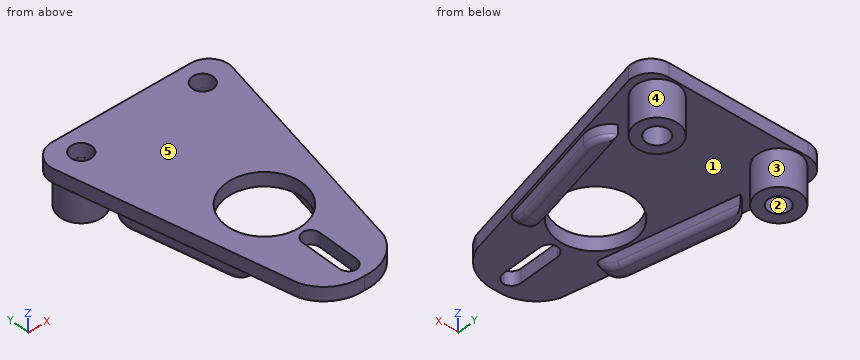
```python
from build123d import *

# Parameters (mm, degrees)
F0_W        = 3.7012519315
F0_H        = 12.7320559695
F0_R        = 8.100129487
F0_R_2      = 2.25
F1_DEPTH    = 3
F2_T1_DEPTH = 3
F3_R        = 4.5649895604
F3_R_2      = 2.4116141927
F3_R_3      = 2.2420485947
F4_DEPTH    = 8
F6_DEPTH    = 3
F7_T1_DEPTH = 14.95289459
F7_T3_DEPTH = 26.4498235383
F7_T5_DEPTH = 26.4498235383
F8_R        = 1


# Not quite as in the source:
# - a fillet or chamfer that OpenCascade refuses, or shapes differently, is made with other operations: its cross-section is extruded or revolved along the edge and cut away or added


with BuildPart() as f1:
    # F0 (on Top) → F1 (new body)
    with BuildSketch(Plane.XY):
        with BuildLine():
            Line((14.8444259539, 34.1621562839), (0, 34.1621562839))
            Line((0, 34.1621562839), (-14.8444259539, 34.1621562839))
            ThreePointArc((-14.8444259539, 34.1621562839), (-18.1303110964, 32.6596806941), (-19.1433615983, 29.1915107518))
            Line((-19.1433615983, 29.1915107518), (-9.0677291155, -18.3654725552))
            ThreePointArc((-9.0677291155, -18.3654725552), (-5.4543132889, -22.6555173257), (0, -23.9638462663))
            ThreePointArc((0, -23.9638462663), (5.4543132889, -22.6555173257), (9.0677291155, -18.3654725552))
            Line((9.0677291155, -18.3654725552), (19.1433615983, 29.1915107518))
            ThreePointArc((19.1433615983, 29.1915107518), (18.1303110964, 32.6596806941), (14.8444259539, 34.1621562839))
        make_face()
        with Locations((0, -15.5778131448)):
            Rectangle(F0_W, F0_H, mode=Mode.SUBTRACT)
        Circle(F0_R, mode=Mode.SUBTRACT)
        with Locations((-13, 29.2403830344)):
            Circle(F0_R_2, mode=Mode.SUBTRACT)
        with Locations((13, 29.2403830344)):
            Circle(F0_R_2, mode=Mode.SUBTRACT)
    extrude(amount=F1_DEPTH)

    # F2: fillet of radius 2 on 4 edges, made by hand

    # F2_s2 → F2_t1 (join)
    with BuildSketch(Plane.XY):
        with BuildLine():
            ThreePointArc((0.1493740343, -9.21178516), (-1.2648395281, -9.7975715976), (-1.8506259657, -11.21178516))
            Line((-1.8506259657, -11.21178516), (-1.8506259657, -9.21178516))
            Line((-1.8506259657, -9.21178516), (0.1493740343, -9.21178516))
        make_face()
        with BuildLine():
            ThreePointArc((1.8506259657, -11.21178516), (1.2648395281, -9.7975715976), (-0.1493740343, -9.21178516))
            Line((-0.1493740343, -9.21178516), (1.8506259657, -9.21178516))
            Line((1.8506259657, -9.21178516), (1.8506259657, -11.21178516))
        make_face()
        with BuildLine():
            ThreePointArc((-1.8506259657, -19.9438411295), (-1.2648395281, -21.3580546919), (0.1493740343, -21.9438411295))
            Line((0.1493740343, -21.9438411295), (-1.8506259657, -21.9438411295))
            Line((-1.8506259657, -21.9438411295), (-1.8506259657, -19.9438411295))
        make_face()
        with BuildLine():
            ThreePointArc((1.8506259657, -19.9438411295), (1.2648395281, -21.3580546919), (-0.1493740343, -21.9438411295))
            Line((-0.1493740343, -21.9438411295), (1.8506259657, -21.9438411295))
            Line((1.8506259657, -21.9438411295), (1.8506259657, -19.9438411295))
        make_face()
    extrude(amount=F2_T1_DEPTH)

    # F3 (on face) → F4 (join)
    with BuildSketch(Plane(origin=(0, 0, 0), x_dir=(1, 0, 0), z_dir=(0, 0, -1))):
        with Locations((13, -29.2403830344)):
            Circle(F3_R)
        with Locations((13, -29.2403830344)):
            Circle(F3_R_2, mode=Mode.SUBTRACT)
        with Locations((-13, -29.2403830344)):
            Circle(F3_R)
        with Locations((-13, -29.2403830344)):
            Circle(F3_R_3, mode=Mode.SUBTRACT)
    extrude(amount=F4_DEPTH)

    # F5 (on face) → F6 (join)
    with BuildSketch(Plane(origin=(0, 0, 0), x_dir=(1, 0, 0), z_dir=(0, 0, -1))):
        Polygon((-7.118105705, 8.1281888095), (-10.5773922314, 8.8652892849), (-16.5612712118, -19.2176554765), (-13.1019846854, -19.9547559519), align=None)
        Polygon((16.5612712118, -19.2176554765), (10.5773922314, 8.8652892849), (7.118105705, 8.1281888095), (13.1019846854, -19.9547559519), align=None)
    extrude(amount=F6_DEPTH)

    # F7: fillet of radius 5 on 4 edges, made by hand

    # F7_s2 → F7_t1 (cut)
    with BuildSketch(Plane.XY.offset(-14.95289459)):
        with BuildLine():
            ThreePointArc((-13.1019846854, 19.9547559519), (-15.2257590624, 17.6540998095), (-15.5648763993, 14.5414745957))
            Line((-15.5648763993, 14.5414745957), (-16.5612712118, 19.2176554765))
            Line((-16.5612712118, 19.2176554765), (-13.1019846854, 19.9547559519))
        make_face()
        with BuildLine():
            ThreePointArc((15.5648763993, 14.5414745957), (15.2257590624, 17.6540998095), (13.1019846854, 19.9547559519))
            Line((13.1019846854, 19.9547559519), (16.5612712118, 19.2176554765))
            Line((16.5612712118, 19.2176554765), (15.5648763993, 14.5414745957))
        make_face()
    extrude(amount=F7_T1_DEPTH, mode=Mode.SUBTRACT)

    # F7_s4 → F7_t3 (cut)
    with BuildSketch(Plane(origin=(23.1298700172, -4.9284839674, 0), x_dir=(0, 0, 1), z_dir=(-0.9780436123, 0.2084003178, 0))):
        with BuildLine():
            ThreePointArc((0, -6.4663076535), (-2.1833001327, -4.622344746), (-3, -1.8837319585))
            Line((-3, -1.8837319585), (-3, -6.4663076535))
            Line((-3, -6.4663076535), (0, -6.4663076535))
        make_face()
    extrude(amount=F7_T3_DEPTH, mode=Mode.SUBTRACT)

    # F7_s6 → F7_t5 (cut)
    with BuildSketch(Plane(origin=(2.7392109406, 0.5836676641, 0), x_dir=(0, 0, 1), z_dir=(-0.9780436123, -0.2084003178, 0))):
        with BuildLine():
            ThreePointArc((0, -6.4663076535), (-2.1833001327, -4.622344746), (-3, -1.8837319585))
            Line((-3, -1.8837319585), (-3, -6.4663076535))
            Line((-3, -6.4663076535), (0, -6.4663076535))
        make_face()
    extrude(amount=F7_T5_DEPTH, mode=Mode.SUBTRACT)

    # F8
    f8_edges = [f1.edges().sort_by_distance(p)[0] for p in [
        (-10.58755, 8.154263, -3),
        (10.58755, 8.154263, -3),
        (13.548639, 5.079072, -3),
        (-13.548639, 5.079072, -3),
        (-15.225759, 17.6541, -3),
        (-10.961675, -7.061813, -2.1833),
        (-7.502388, -6.324713, -2.1833),
        (15.225759, 17.6541, -3),
        (7.502388, -6.324713, -2.1833),
        (10.961675, -7.061813, -2.1833),
    ]]
    fillet(f8_edges, radius=F8_R)


solid = f1.part
```
Geometry check sheet. Reference: the model listing, model coordinates, mm. Face numbers are marked on the shaded views. A direction names the side the tool comes from. Coordinates: 2 decimals unless noted, no trailing zeros. Order: outer loops, then holes, each group sorted by start corner. A loop starts at its lowest first (then second) coordinate and runs counter-clockwise, first axis right, second up. Notation, with made-up numbers: M 6.5,19 L 47.5,19 A20 cw 47.5,56 Z; hole C -33.5,17.5 d7. An arc over 180 degrees is marked long. One line per question, with ' | ' between items. Start each with the question number.
Item 1: Draft check along X on the marked faces 3, 4 and 5. Enter one of: pulls with the +X half, pulls with the -X half, needs draft (parallel to the pull), parting line crosses it, or undercut.
Item 2: Gauge pin test, flat ends, axial feed: pin 1 (2 mm diameter, centred on y = 12.5, z = -5.5, fed in from +X); pin 2 (1.7 mm diameter, centred on x = -12.5, y = 3.5, fed in from -Z); pin 3 (4 mm diameter, centred on x = -14.5, z = -7, fed in from -Y); pin 4 (2.5 mm diameter, centred on y = -13.5, z = 2, fed in from -X). Record the tip position at first contact, or that the pin passes through.
Item 3: Cross-section at A-A on y = -14.5. Enter the section's corners in (x, z).
Item 4: Cross-section at B-B on z = -5.5. Enter the section's corners in (x, y), then the cut area to 3 significant figures.
Item 5: Set-up check for the marked faces 1 and 2: record each of +Z, -Z, +X, -X, +Y, -Y from which the full face is reachable in a straight line by a thin tool's end or side.
Item 6: Material ranges on L1, parallel to Y at x = -13, z = -4.25; L2, parallel to Z at x = -12.5, y = 13; L3, parallel to Z at x = 0, y = 24.5, recorded low to high. Write a range as [from, to].
Findings:
1) face 3: undercut | face 4: undercut | face 5: needs draft
2) pin 1: passes through | pin 2: stops at z = -3 | pin 3: stops at y = 24.68 | pin 4: stops at x = -10.36
3) outline: M -9.89,0 L -1.85,0 L -1.85,3 L -9.89,3 Z; M 1.85,0 L 9.89,0 L 9.89,3 L 1.85,3 Z
4) outline: C -13,29.24 d9.13; C 13,29.24 d9.13; hole C -13,29.24 d4.48; hole C 13,29.24 d4.82 | area: 96.9 mm²
5) face 1: -Z | face 2: +Z, -Z
6) L1: y = [24.68, 27], [31.48, 33.81] | L2: z = [-2.99, 3] | L3: z = [0, 3]
